Check sheet for the modelled part. Datum: model origin and axes. Units: mm. A direction names the side the tool comes from. Give positions to 0.01 mm unless a question says otherwise; leave off trailing zeros. Order: outer loops, then holes, each group sorted by start corner. A loop starts at its lowest first (then second) coordinate and runs counter-clockwise, first axis right, second up. Notation, with made-up numbers: (38, -20.75) -> (80, -20.75) arc R19 ccw to (80, -4.75) -> close; hole circle Ø1 at (87.25, 24.5). An arc over 180 degrees is marked (long way). One line per question, with ' | ' between items.
Autodesk Inventor part; units mm, degrees
ref_plane "YZ Plane" through (0, 0, 0) normal (1, 0, 0) x (0, 1, 0)
ref_plane "XZ Plane" through (0, 0, 0) normal (0, 1, 0) x (-1, 0, 0)
ref_plane "XY Plane" through (0, 0, 0) normal (0, 0, 1) x (1, 0, 0)
sketch "Sketch1" plane through (0, 0, 0) normal (0, 1, 0) x (-1, 0, 0)
  line L0 (-5, 5) -> (5, 5)
  line L1 (5, 5) -> (5, -5)
  line L2 (5, -5) -> (-5, -5)
  line L3 (-5, -5) -> (-5, 5)
  line L4 (-5, 5) -> (5, -5) construction
  line L5 (5, 5) -> (-5, -5) construction
  point P0 (0, 0)
  dimension "d0" = 10
  dimension "d1" = 10
extrude "Extrusion1" add sketch "Sketch1" along normal blind 1.5
sketch "Sketch2" plane through (0, 1.5, 0) normal (0, 1, 0) x (1, 0, 0)
  line L0 (-5, -5) -> (-3.5, -5)
  line L1 (-5, -5) -> (5, -5)
  line L2 (-3.5, -5) -> (-3.5, 3.5)
  line L3 (-3.5, 3.5) -> (5, 3.5)
  line L4 (5, 3.5) -> (5, 5)
  line L5 (5, 5) -> (-5, 5)
  line L6 (-5, 5) -> (-5, -5)
  point P0 (0, 0)
  dimension "d4" = 1.5
  dimension "d5" = 8.5
  dimension "d6" = 90
  dimension "d7" = 8.5
  dimension "d8" = 90
  dimension "d9" = 10
  dimension "d10" = 90
extrude "Extrusion2" add sketch "Sketch2" along normal blind 8.5
sketch "Sketch3" plane through (0, 1.5, 0) normal (0, 1, 0) x (1, 0, 0)
  circle A0 centre (0.8, 3.1) radius 0.5
  line L0 (5, 3.5) -> (-3.5, 3.5)
  line L1 (-3.5, 3.5) -> (-3.5, -5)
  point P0 (0, 0)
  dimension "d13" = 1
  dimension "d14" = 0.4
  dimension "d15" = 4.3
extrude "Extrusion3" cut sketch "Sketch3" against normal blind 8.5
sketch "Sketch4" plane through (-3.5, 1.5, -3.5) normal (0, 0, 1) x (1, 0, 0)
  circle A0 centre (1, 3.7) radius 0.5
  line L0 (8.5, 0) -> (0, 0)
  line L1 (0, 0) -> (0, 8.5)
  point P0 (3.5, -1.5)
  dimension "d18" = 1
  dimension "d19" = 3.7
  dimension "d20" = 1
extrude "Extrusion4" cut sketch "Sketch4" against normal blind 8.5
sketch "Sketch5" plane through (0, 0, 0) normal (0, -1, 0) x (1, 0, 0)
  circle A0 centre (0.8, -3.1) radius 0.5
  circle A1 centre (0.8, -3.1) radius 0.5
  point P0 (0, 0)
  dimension "d23" = 1
  dimension "d24" = 0
extrude "Extrusion5" cut sketch "Sketch5" against normal blind 10
sketch "Sketch6" plane through (-3.5, 1.5, 5) normal (1, 0, 0) x (0, 0, -1)
  circle A0 centre (4.8, 1) radius 0.5
  line L0 (0, 0) -> (8.5, 0)
  line L1 (8.5, 0) -> (8.5, 8.5)
  point P0 (5, -1.5)
  dimension "d27" = 1
  dimension "d28" = 1
  dimension "d29" = 3.7
extrude "Extrusion6" cut sketch "Sketch6" against normal blind 2
sketch "Sketch7" plane through (-5, 0, 5) normal (0, 0, 1) x (1, 0, 0)
  line L0 (0, 0) -> (10, 0)
  line L1 (10, 0) -> (10, 10)
  line L2 (10, 10) -> (0, 10)
  line L3 (0, 10) -> (0, 0)
  point P0 (5, 0)
extrude "Extrusion7" cut sketch "Sketch7" against normal blind 3
sketch "Sketch8" plane through (-5, 0, 2) normal (0, 0, 1) x (1, 0, 0)
  line L0 (0, 0) -> (10, 0)
  line L1 (10, 0) -> (10, 10)
  line L2 (10, 10) -> (0, 10)
  line L3 (0, 10) -> (0, 0)
  point P0 (5, 0)
extrude "Extrusion8" add sketch "Sketch8" along normal blind 1.5
sketch "Sketch9" plane through (-5, 0, 3.5) normal (0, 0, 1) x (1, 0, 0)
  circle A0 centre (6, 6) radius 1
  line L0 (0, 0) -> (10, 0)
  line L1 (0, 10) -> (0, 0)
  point P0 (5, 0)
  dimension "d36" = 2
  dimension "d37" = 6
  dimension "d38" = 6
extrude "Extrusion9" cut sketch "Sketch9" against normal blind 1.5
properties part number "Corner2"
Q1. Section check C-C (x = -2.5). Enter the section's corners in (y, z).
Result sheet:
outline: (0, -5) -> (4.7, -5) -> (4.7, -3.5) -> (1.5, -3.5) -> (1.5, 2) -> (10, 2) -> (10, 3.5) -> (0, 3.5) -> close; (5.7, -5) -> (10, -5) -> (10, -3.5) -> (5.7, -3.5) -> close
Q2. Section check B-B (y = 2.5). Enter the section's corners in (x, z).
Result sheet:
outline: (-5, -5) -> (5, -5) -> (5, -3.5) -> (1.1, -3.5) arc R0.5 cw to (0.5, -3.5) -> (-3.5, -3.5) -> (-3.5, -0.3) -> (-5, -0.3) -> close; (-5, 0.7) -> (-3.5, 0.7) -> (-3.5, 2) -> (5, 2) -> (5, 3.5) -> (-5, 3.5) -> close
Q3. Thickness scan on line 1 (Z direction, x = 0.75, y = 5); line 2 (Z direction, x = -2, y = 9.5); line 3 (Y direction, x = 1, z = 2.4). Record the ranges inside material, lowest first.
Result sheet:
line 1: z = -5 to -3.6, 2 to 3.5 | line 2: z = -5 to -3.5, 2 to 3.5 | line 3: y = 0 to 5, 7 to 10
Q4. Section check A-A (z = -3.1). Enter the section's corners in (x, y), and give its area (4 significant figures).
Result sheet:
outline: (-5, 0) -> (0.3, 0) -> (0.3, 1.5) -> (-3.5, 1.5) -> (-3.5, 10) -> (-5, 10) -> close; (1.3, 0) -> (5, 0) -> (5, 1.5) -> (1.3, 1.5) -> close | area: 26.25 mm2
Q5. Section check D-D (y = 5.2). Enter the section's corners in (x, z).
Result sheet:
outline: (-5, -5) -> (-3, -5) -> (-3, -3.5) -> (-3.5, -3.5) -> (-3.5, 2) -> (0.4, 2) -> (0.4, 3.5) -> (-5, 3.5) -> close; (-2, -5) -> (5, -5) -> (5, -3.5) -> (1.1, -3.5) arc R0.5 cw to (0.5, -3.5) -> (-2, -3.5) -> close; (1.6, 2) -> (5, 2) -> (5, 3.5) -> (1.6, 3.5) -> close
Q6. Access from +Z, -Z, +X, -X, +Y, -Y to the whole of each face (thin tool, end or side, straight path). Record for faces 5 (the face through (-0.3, 5.8, 2)), 6 (the face through (0, 5, 3.5)), 7 (the face through (-4.24, 2.996, 0.265)), 8 (the face through (1, 7, 3)), 9 (the face through (-2.565, 5.696, -4.24)).
Result sheet:
face 5: +X, +Y | face 6: +Z, +X, -X, +Y, -Y | face 7: +X, -X | face 8: +Z | face 9: -Z
Q7. Depth check by flat-ended pin: pin 1 Ø5 at (y, z) = (7.5, -2.5) entering from +X; pin 2 Ø3 at (y, z) = (5.5, -1.5) entering from +X; pin 3 Ø1.6 at (x, z) = (-0.5, -1) entering from +Y. Enter the tip coordinate at first touch or a pass-through.
Result sheet:
pin 1: stops at x = 5 | pin 2: stops at x = -3.5 | pin 3: stops at y = 1.5
Q8. Mould release check, pull along Z, two halves, no side actions. Record for faces 1 (the face through (-5, 5, -1)), 2 (the face through (1, 1.5, -1)), 3 (the face through (-3.5, 6, -1)), 4 (the face through (0, 5, -5)): pulls with the +Z half, pulls with the -Z half, needs draft (parallel to the pull), parting line crosses it, or undercut.
Result sheet:
face 1: needs draft | face 2: undercut | face 3: undercut | face 4: pulls with the -Z half
